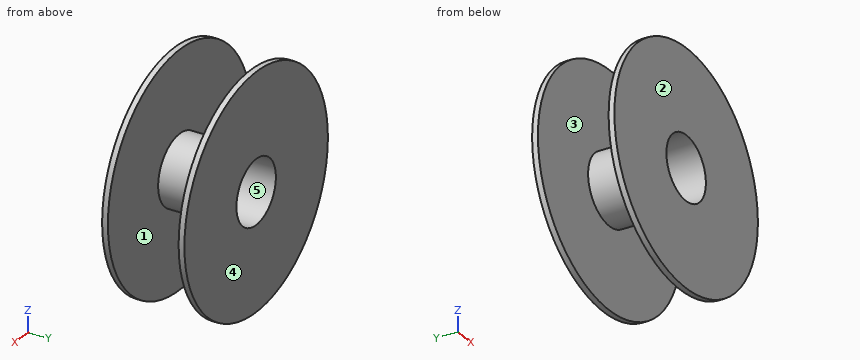
from build123d import *

# Parameters (mm, degrees)
F0_R        = 100
F0_R_2      = 30
F1_DEPTH    = 5
F2_START    = 61
F1_FACE_R   = 100
F1_FACE_R_2 = 30
F2_DEPTH    = 5
F0_R_3      = 27.5
F3_DEPTH    = 71


with BuildPart() as f1:
    # F0 (on Front) → F1 (new body)
    with BuildSketch(Plane.XZ):
        Circle(F0_R)
        Circle(F0_R_2, mode=Mode.SUBTRACT)
    extrude(amount=-F1_DEPTH)



with BuildPart() as f2:
    # F1_face (on face) → F2 (new body)
    with BuildSketch(Plane(origin=(0, 5, 0), x_dir=(1, 0, 0), z_dir=(0, 1, 0)).offset(F2_START)):
        Circle(F1_FACE_R)
        Circle(F1_FACE_R_2, mode=Mode.SUBTRACT)
    extrude(amount=F2_DEPTH)


with BuildPart() as f1_1:
    add(f1.part)

    add(f2.part)  # F3 merges F2
    # F0 (on Front) → F3 (join)
    with BuildSketch(Plane.XZ):
        Circle(F0_R_2)
        Circle(F0_R_3, mode=Mode.SUBTRACT)
    extrude(amount=-F3_DEPTH)


solid = f1_1.part
The listing builds one solid part. Answer for the finished solid, in the listing's coordinates (mm). Face numbers are marked on the shaded views. A direction names the side the tool comes from. Round coordinates to 2 decimals unless told otherwise and drop trailing zeros. Loops run counter-clockwise (first coordinate to the right, second up) from the corner with the lowest first, then second, coordinate; pieces in that order, holes last. Notation, with made-up numbers: M -12,52 L 19,52 A23 ccw 19,84 Z; hole C 1.25,28 d11. An arc over 180 degrees is marked long. Return JSON: item names as keys, results as strings.
Q1. Find the intervals of material crossed by line 1 along Y through (x, z) = (-67.5, -20.5); line 2 along Z through (x, y) = (0, 41); line 3 along X through (y, z) = (11.5, 5.5), in increasing order. Write a range as from..to.
Results list:
{"line 1": "y = 0..5, 66..71", "line 2": "z = -30..-27.5, 27.5..30", "line 3": "x = -29.49..-26.94, 26.94..29.49"}
Q2. The mould has two halves that part along Y. Classify the marked faces 3, 4 and 5: released by +Y, released by -Y, zero draft, split by the parting line, or undercut.
Results list:
{"face 3": "undercut", "face 4": "released by +Y", "face 5": "zero draft"}
Q3. Find section D-D, the plane z = 65. Determine the outline of the cut face in (x, y), plus the area to 3 significant figures.
Results list:
{"outline": "M -75.99,0 L 75.99,0 L 75.99,5 L -75.99,5 Z; M -75.99,66 L 75.99,66 L 75.99,71 L -75.99,71 Z", "area": "1,520 mm2"}
Q4. Find section B-B, the plane x = 0. Determine the outline of the cut face in (y, z), plus the area to 4 significant figures.
Results list:
{"outline": "M 0,-100 L 5,-100 L 5,-30 L 66,-30 L 66,-100 L 71,-100 L 71,-27.5 L 0,-27.5 Z; M 0,27.5 L 71,27.5 L 71,100 L 66,100 L 66,30 L 5,30 L 5,100 L 0,100 Z", "area": "1,755 mm2"}
Q5. Each of these flat-tipped pins is pushed along its axis until it touches: pin 1 Ø5 at (x, z) = (19.5, -13) entering from -Y; pin 2 Ø1 at (y, z) = (10.5, -14.5) entering from +X; pin 3 Ø12 at (y, z) = (28.5, 27.5) entering from +X. Where does it stop, or does it pass through?
Results list:
{"pin 1": "passes through", "pin 2": "stops at x = 26.53", "pin 3": "stops at x = 20.92"}
Q6. Find section A-A, the plane z = 0. Determine the outline of the cut face in (x, y).
Results list:
{"outline": "M -100,0 L -27.5,0 L -27.5,71 L -100,71 L -100,66 L -30,66 L -30,5 L -100,5 Z; M 27.5,0 L 100,0 L 100,5 L 30,5 L 30,66 L 100,66 L 100,71 L 27.5,71 Z"}
Q7. Find section C-C, the plane y = 44. Determine the outline of the cut face in (x, z), plus the area to 3 significant figures.
Results list:
{"outline": "C 0,0 d60; hole C 0,0 d55", "area": "452 mm2"}
Q8. Which of the six approach directions +Z, -Z, +X, -X, +Y, -Y give full straight-line access (tool end or side, diameter ignored) to the marked faces 1 and 2?
Results list:
{"face 1": "none", "face 2": "+Z, -Z, +X, -X, -Y"}
